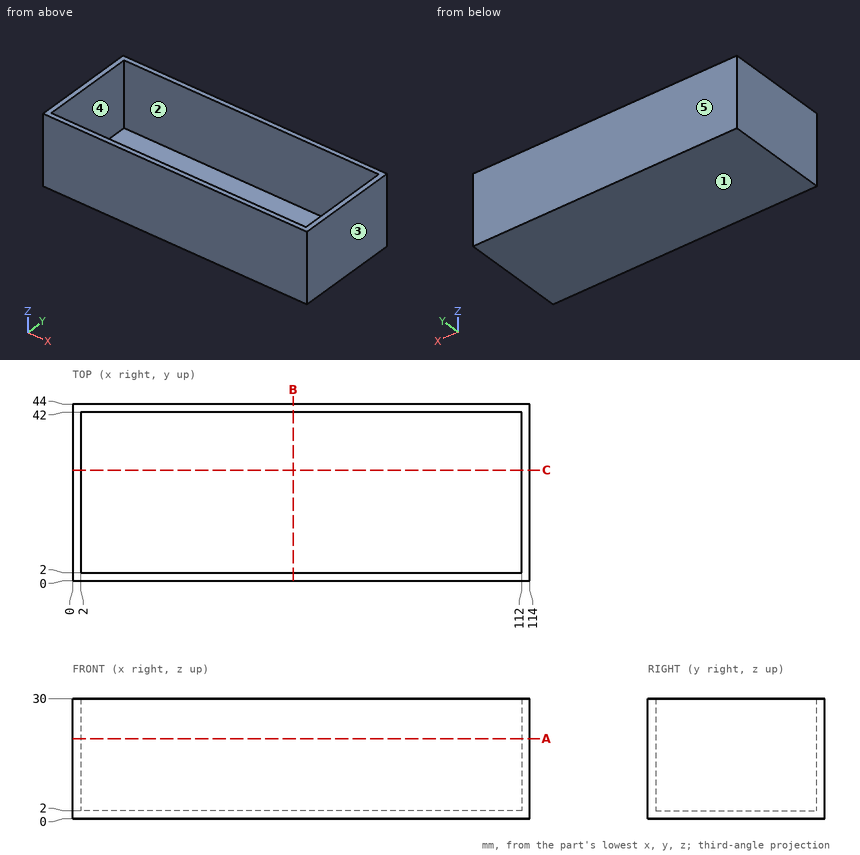
Could you check a few things on this drawing? It's one solid part, dimensions in mm from its lowest x, y, z. A direction names the side the tool comes from. Give positions to 0.01 mm unless a question says otherwise; leave off trailing zeros. Write each loop counter-clockwise with the first axis right and the second up, starting at its lowest first coordinate (ties: lowest second). Pieces come first, ordered by that corner, then holes. Notation, with made-up numbers: (-3.5, -32) -> (50.5, -32) arc R33 cw to (50.5, -2) -> close; hole circle Ø8 at (83.5, 7.5). An arc over 180 degrees is marked (long way). Answer as a JSON object with one key per item and string values.
Q1. Suppose I cut it at C-C on y = 27.5. Write out the boundary of the cut face in (x, z).
Taken from the geometry:
{"outline": "(0, 0) -> (114, 0) -> (114, 30) -> (112, 30) -> (112, 2) -> (2, 2) -> (2, 30) -> (0, 30) -> close"}
Q2. Please list where these lines run through material, in increasing order: L1, parallel to Y at x = 30, z = 27.5; L2, parallel to X at y = 27, z = 28; L3, parallel to Z at x = 94, y = 24.
Taken from the geometry:
{"L1": "y = 0 to 2, 42 to 44", "L2": "x = 0 to 2, 112 to 114", "L3": "z = 0 to 2"}
Q3. Will this pin go through, and if not, where does the flat tip stop? pin 1 Ø1.5 at (x, y) = (49, 19) entering from +Z.
Taken from the geometry:
{"pin 1": "stops at z = 2"}
Q4. Suppose I cut it at B-B on x = 55. Write out the boundary of the cut face in (y, z).
Taken from the geometry:
{"outline": "(0, 0) -> (44, 0) -> (44, 30) -> (42, 30) -> (42, 2) -> (2, 2) -> (2, 30) -> (0, 30) -> close"}
Q5. Which directions (+Z, -Z, +X, -X, +Y, -Y) give clear straight access to the entire face, cutting with the end or side of a thin tool? Please do the marked faces 4 and 5.
Taken from the geometry:
{"face 4": "+Z", "face 5": "+Z, -Z, +X, -X, +Y"}
Q6. We'd pull the mould along X, two halves only. Please class the marked faces 1, 2 and 3: released by +X, released by -X, zero draft, split by the parting line, or undercut.
Taken from the geometry:
{"face 1": "zero draft", "face 2": "undercut", "face 3": "released by +X"}
Q7. Suppose I cut it at A-A on z = 20. Write out the boundary of the cut face in (x, y), then the cut area to 3 significant figures.
Taken from the geometry:
{"outline": "(0, 0) -> (114, 0) -> (114, 44) -> (0, 44) -> close; hole (2, 2) -> (112, 2) -> (112, 42) -> (2, 42) -> close", "area": "616 mm²"}
